```python
from build123d import *

# Parameters (mm, degrees)
EXTRUDE1_DEPTH     = 180
EXTRUDE2_DEPTH     = 115
CUT_EXTRUDE1_DEPTH = 35


with BuildPart() as part:
    # Sketch1 → Extrude1 (new body)
    with BuildSketch(Plane(origin=(0, 0, 0), x_dir=(0, 0, -1), z_dir=(1, 0, 0))):
        Polygon((0, 0), (50, 0), (50, 41.954981559), align=None)
    extrude(amount=EXTRUDE1_DEPTH)

    # Sketch5 → Extrude2 (add)
    with BuildSketch(Plane(origin=(-16.367513459, 0, 28.349364905), x_dir=(0.866025404, 0, 0.5), z_dir=(-0.5, 0, 0.866025404))):
        Polygon((43.301270189, 0), (78.301270189, 24.507263837), (113.301270189, 0), align=None)
    extrude(amount=-EXTRUDE2_DEPTH)

    # Sketch6 → Cut-Extrude1 (cut, symmetric)
    with BuildSketch(Plane(origin=(51.443375673, 0, 67.5), x_dir=(0.5, 0, -0.866025404), z_dir=(0.866025404, 0, 0.5))):
        Polygon((29.206619723, 24.507263837), (0, 24.507263837), (0, 0), align=None)
    extrude(amount=CUT_EXTRUDE1_DEPTH, both=True, mode=Mode.SUBTRACT)


solid = part.part
```
Verification items for the finished model (mm, model axes). A direction names the side the tool comes from. Round coordinates to 2 decimals unless told otherwise and drop trailing zeros. Loops run counter-clockwise (first coordinate to the right, second up) from the corner with the lowest first, then second, coordinate; pieces in that order, holes last. Notation, with made-up numbers: (65, 78.25) -> (102, 78.25) arc R31 ccw to (102, 105.25) -> close; hole circle Ø5 at (74, 25). An arc over 180 degrees is marked (long way). Answer as a JSON object with one key per item and string values.
Q1. Draft check along Z on faces 1 (the flat face through (89, 21, -50)), 2 (the flat face through (93.913, 12.425, 28.451)), 3 (the flat face through (63.6, 12.1, 11)), 4 (the flat face through (0, 12, -36)). Enter one of: pulls with the +Z half, pulls with the -Z half, needs draft (parallel to the pull), parting line crosses it, or undercut.
Data:
{"face 1": "pulls with the -Z half", "face 2": "pulls with the +Z half", "face 3": "undercut", "face 4": "needs draft"}
Q2. Section check D-D (x = 70). Record the boundary of the cut face in (y, z), then the cut area to 3 significant figures.
Data:
{"outline": "(0, -50) -> (41.95, -50) -> (8.56, -10.2) -> (24.51, 35.36) -> (18.34, 52.98) -> (0, 78.21) -> close", "area": "2,370 mm2"}
Q3. Section check C-C (y = 14.5). Record the boundary of the cut face in (x, z), then the cut area to 3 significant figures.
Data:
{"outline": "(0, -50) -> (180, -50) -> (180, -17.28) -> (116.89, -17.28) -> (72.46, 59.68) -> (47.71, 45.39) -> (83.89, -17.28) -> (0, -17.28) -> close", "area": "8,190 mm2"}
Q4. Scan lines: line 1 (Y direction, x = 96, z = -8); line 2 (Y direction, x = 43, z = -14.5); line 3 (Z direction, x = 35, y = 21). Record each from-to range of solid material in increasing order. Write a range as from..to.
Data:
{"line 1": "y = 0..23.92", "line 2": "y = 0..12.17", "line 3": "z = -50..-25.03"}
Q5. Access from +Z, -Z, +X, -X, +Y, -Y to the whole of each face (thin tool, end or side, straight path). Record for faces 5 (the flat face through (88.74, 21.27, -25.35)), 6 (the flat face through (180, 12, -36)).
Data:
{"face 5": "+Y", "face 6": "+Z, -Z, +X, +Y, -Y"}
Q6. Go/stop test with flat-tipped pins: P1, Ø1, axis at x = 94.5, z = 52, coming from the +Y side; P2, Ø12, axis at y = 26.5, z = 45.5, coming from the -X side; P3, Ø6, axis at x = 44.5, z = 21.5, coming from the +Y side. Record where each tip stops, or that it passes through.
Data:
{"P1": "stops at y = 4.17", "P2": "stops at x = 59.43", "P3": "stops at y = 6.29"}
Q7. Section check A-A (x = 32). Record the boundary of the cut face in (y, z), then the cut area to 3 significant figures.
Data:
{"outline": "(0, -50) -> (41.95, -50) -> (0, 0) -> close; (0, 31.18) -> (5.93, 48.11) -> (0, 56.27) -> close", "area": "1,120 mm2"}
Q8. Section check B-B (z = -19). Record the boundary of the cut face in (x, y).
Data:
{"outline": "(0, 0) -> (180, 0) -> (180, 15.94) -> (115.51, 15.94) -> (101.38, 24.51) -> (87.26, 15.94) -> (0, 15.94) -> close"}
